from build123d import *

# Parameters (mm, degrees)
EXTRUDE_2_DEPTH          = 10
SKETCH_3_R               = 1.65
CUT_EXTRUDE_1_DEPTH      = 76
CUT_EXTRUDE_1_DEPTH_BACK = 6
EXTRUDE_3_DEPTH          = 2
MIRROR_2_COPY_1_DEPTH    = 2


with BuildPart() as part:
    # 草图1 → 凸台-拉伸2 (new body)
    with BuildSketch(Plane.XY):
        Polygon((-40, 0), (40, 0), (40, -11), (35, -11), (35, -5), (-35, -5), (-35, -11), (-40, -11), align=None)
    extrude(amount=EXTRUDE_2_DEPTH)

    # 草图3 → 切除-拉伸1 (cut, two sides)
    with BuildSketch(Plane(origin=(-35, 0, 0), x_dir=(0, 0, -1), z_dir=(1, 0, 0))) as cut_extrude_1_sk:
        with Locations((-5, -8)):
            Circle(SKETCH_3_R)
    extrude(amount=CUT_EXTRUDE_1_DEPTH, mode=Mode.SUBTRACT)
    extrude(cut_extrude_1_sk.sketch, amount=-CUT_EXTRUDE_1_DEPTH_BACK, mode=Mode.SUBTRACT)

    # 草图4 → 凸台-拉伸3 (add)
    with BuildSketch(Plane(origin=(0, 0, 0), x_dir=(-1, 0, 0), z_dir=(0, 0, -1))):
        Polygon((29, -5), (35, -11), (35, -5), align=None)
    extrude_3 = extrude(amount=-EXTRUDE_3_DEPTH)

    # 镜向1: 凸台-拉伸3 across plane
    add(extrude_3.mirror(Plane.XY.offset(5)))

    # 镜向2: 凸台-拉伸3 across plane
    add(extrude_3.mirror(Plane(origin=(0, 0, 0), x_dir=(0, 0, 1), z_dir=(1, 0, 0))))

    # 镜向2 copy 1 sketch → 镜向2 copy 1 (add)
    with BuildSketch(Plane.XY.offset(10)):
        Polygon((29, -5), (35, -11), (35, -5), align=None)
    extrude(amount=-MIRROR_2_COPY_1_DEPTH)


solid = part.part
The listing builds one solid part. Answer for the finished solid, in the listing's coordinates (mm). A direction names the side the tool comes from. Coordinates: 2 decimals unless noted, no trailing zeros. Write each loop counter-clockwise with the first axis right and the second up, starting at its lowest first coordinate (ties: lowest second). Pieces come first, ordered by that corner, then holes. Notation, with made-up numbers: M 69,18 L 103,18 A22 cw 103,31 Z; hole C 11,72 d5. An arc over 180 degrees is marked long. Write each question's results on one line, items separated by ' | '.
Item 1: The part is cut by section A-A on z = 5. Determine the outline of the cut face in (x, y).
Answer below:
outline: M -40,-11 L -35,-11 L -35,-9.65 L -40,-9.65 Z; M -40,-6.35 L -35,-6.35 L -35,-5 L 35,-5 L 35,-6.35 L 40,-6.35 L 40,0 L -40,0 Z; M 35,-11 L 40,-11 L 40,-9.65 L 35,-9.65 Z
Item 2: Given P1, Ø1.8, axis at x = -31.5, y = -9, coming from the +Z side; P2, Ø6.5, axis at x = 31, y = -8.5, coming from the -Z side; P3, Ø4, axis at x = -21, z = 6, coming from the -Y side, each flat-ended and moving along its own axis, determine where each tip first touches the part or whether it passes through.
Answer below:
P1: through | P2: z = 0 | P3: y = -5
Item 3: Consider probe 1 along Z at (x, y) = (37, -8); probe 2 along Y at (x, z) = (38.6, 5); probe 3 along X at (y, z) = (-6, 4). Determine where each line is inside the solid, lowest interval first. Write a range as [from, to].
Answer below:
probe 1: [0, 3.35], [6.65, 10] | probe 2: [-11, -9.65], [-6.35, 0] | probe 3: [-40, -35], [35, 40]
Item 4: For a pull along Y with two mould halves and no side action, classify faces 4 (the face through (37.47, -7.93, 6.65)), 5 (the face through (-1, 0, 5)), 6 (the face through (32, -8, 9)) as released by +Y, released by -Y, zero draft, split by the parting line, or undercut.
Answer below:
face 4: undercut | face 5: released by +Y | face 6: released by -Y
Item 5: The part is cut by section B-B on y = -8. Determine the outline of the cut face in (x, z).
Answer below:
outline: M -40,0 L -32,0 L -32,2 L -35,2 L -35,3.35 L -40,3.35 Z; M -40,6.65 L -35,6.65 L -35,8 L -32,8 L -32,10 L -40,10 Z; M 32,0 L 40,0 L 40,3.35 L 35,3.35 L 35,2 L 32,2 Z; M 32,8 L 35,8 L 35,6.65 L 40,6.65 L 40,10 L 32,10 Z
Item 6: The part is cut by section C-C on x = 1. Determine the outline of the cut face in (y, z).
Answer below:
outline: M -5,0 L 0,0 L 0,10 L -5,10 Z
Item 7: Which of the six approach directions +Z, -Z, +X, -X, +Y, -Y give full straight-line access (tool end or side, diameter ignored) to faces 1 (the face through (40, -5, 5)), 2 (the face through (32, -8, 1)), 3 (the face through (-33, -7, 8))?
Answer below:
face 1: +Z, -Z, +X, +Y, -Y | face 2: +Z, -Z, -Y | face 3: -Y
